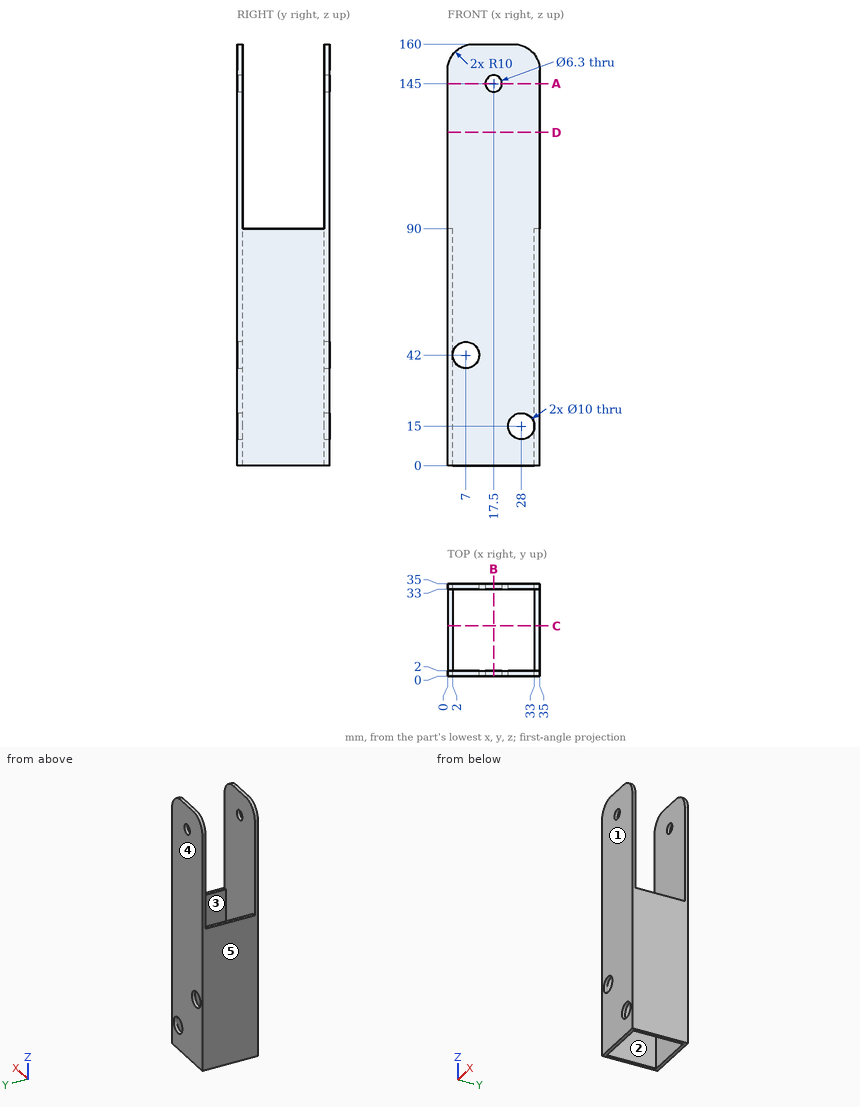
Part print with two shaded views. Sizes in mm from the minimum x, y, z corner. A direction names the side the tool comes from. Coordinates: 2 decimals unless noted, no trailing zeros. Write each loop counter-clockwise with the first axis right and the second up, starting at its lowest first coordinate (ties: lowest second). Pieces come first, ordered by that corner, then holes. Notation, with made-up numbers: (86, 1.25) - (135, 1.25) arc R33 ccw to (135, 36.25) - close; hole circle Ø6 at (-23, -14.5). An arc over 180 degrees is marked (long way). Put each result on its own line as item: value.
1. Probe line 1 along X through (y, z) = (34, 145); line 2 along Y through (x, z) = (21, 11); line 3 along X through (y, z) = (1.6, 42). List the from-to ranges inside material, lowest first. Write a range as [from, to].
Final values:
line 1: x = [0, 14.35], [20.65, 35]
line 2: y = [0, 2], [33, 35]
line 3: x = [0, 2], [12, 35]
2. Flat gauge pins, fed straight in: pin 1 Ø0.6 at (x, y) = (1, 18.5) entering from +Z; pin 2 Ø5.5 at (x, z) = (17.5, 145) entering from +Y. Where does each tip first touch, or does it go through?
Final values:
pin 1: stops at z = 90
pin 2: passes through
3. 3-axis set-ups, long thin cutter, end or side, ignore diameter. For the marked faces 1 and 2: which of +Z, -Z, +X, -X, +Y, -Y reach the whole face in a straight line?
Final values:
face 1: +Z, -Z, +X, -X, -Y
face 2: +Z, -Z
4. Band-saw the part on D-D (z = 126.5). Write the cut outline in (x, y).
Final values:
outline: (0, 0) - (35, 0) - (35, 2) - (0, 2) - close; (0, 33) - (35, 33) - (35, 35) - (0, 35) - close
5. Two-plate mould, pull along X, no slides. Class the marked faces 3, 4 and 5: +X half, -X half, draft (parallel to the pull), parting line (faces both ways), or undercut.
Final values:
face 3: undercut
face 4: draft
face 5: -X half
6. Band-saw the part on C-C (y = 19). Write the cut outline in (x, z), then the cut area to 3 significant figures.
Final values:
outline: (0, 0) - (2, 0) - (2, 90) - (0, 90) - close; (33, 0) - (35, 0) - (35, 90) - (33, 90) - close
area: 360 mm²
7. Band-saw the part on B-B (x = 17.5). Write the cut outline in (y, z), then the cut area to 3 significant figures.
Final values:
outline: (0, 0) - (2, 0) - (2, 141.85) - (0, 141.85) - close; (0, 148.15) - (2, 148.15) - (2, 160) - (0, 160) - close; (33, 0) - (35, 0) - (35, 141.85) - (33, 141.85) - close; (33, 148.15) - (35, 148.15) - (35, 160) - (33, 160) - close
area: 615 mm²
8. Band-saw the part on A-A (z = 145). Write the cut outline in (x, y).
Final values:
outline: (0, 0) - (14.35, 0) - (14.35, 2) - (0, 2) - close; (0, 33) - (14.35, 33) - (14.35, 35) - (0, 35) - close; (20.65, 0) - (35, 0) - (35, 2) - (20.65, 2) - close; (20.65, 33) - (35, 33) - (35, 35) - (20.65, 35) - close
